```python
from build123d import *

# Parameters (mm, degrees)
BOX_W           = 18
BOX_H           = 200
BOX_DEPTH       = 137
SKETCH001_W     = 18
SKETCH001_H     = 137
POCKET001_DEPTH = 5
SKETCH003_R     = 1.55
HOLE_DEPTH      = 13.001


with BuildPart() as body002:
    # Box → Box (new body)
    with BuildSketch(Plane.XY):
        with Locations((9, 100)):
            Rectangle(BOX_W, BOX_H)
    extrude(amount=BOX_DEPTH)

    # Sketch001 (on Face2 of BaseFeature001) → Pocket001 (cut)
    with BuildSketch(Plane.YZ.offset(18)):
        with Locations((141, 68.5)):
            Rectangle(SKETCH001_W, SKETCH001_H)
    extrude(amount=-POCKET001_DEPTH, mode=Mode.SUBTRACT)

    # Sketch003 (on Face9 of Pocket001) → Hole (cut, through all)
    with BuildSketch(Plane.YZ.offset(13)):
        with Locations((141, 97)):
            Circle(SKETCH003_R)
        with Locations((141, 57)):
            Circle(SKETCH003_R)
        with Locations((141, 17)):
            Circle(SKETCH003_R)
    extrude(amount=-HOLE_DEPTH, mode=Mode.SUBTRACT)


with BuildPart() as rightleg:
    # Part__Mirroring: instance of Body002
    add(body002.part.mirror(Plane(origin=(0, 0, 0), x_dir=(0, -1, 0), z_dir=(1, 0, 0))))


with BuildPart() as rightleg_1:
    # Part__Mirroring placement: moved
    add(rightleg.part.moved(Location((350, 0, 0))))


solid = rightleg_1.part
```
The model under review builds one solid part; all positions refer to its coordinate system, in mm. A direction names the side the tool comes from. Give positions to 0.01 mm unless a question says otherwise; leave off trailing zeros. Write each loop counter-clockwise with the first axis right and the second up, starting at its lowest first coordinate (ties: lowest second). Pieces come first, ordered by that corner, then holes. Notation, with made-up numbers: (45.25, 60) -> (67.25, 60) arc R19 cw to (67.25, 66) -> close; hole circle Ø11 at (52.25, 38.25). An arc over 180 degrees is marked (long way). Answer in a Markdown table with one row per item.
1) Tool access review of faces 1 (the flat face through (341, 200, 68)), 2 (the flat face through (337, 141, 69)): name each direction out of +Z, -Z, +X, -X, +Y, -Y from which nothing blocks a thin tool from reaching the whole face with its end or side.
Worked answers:
| item | result |
|---|---|
| face 1 | +Z, -Z, +X, -X, +Y |
| face 2 | +Z, -Z, -X |
2) Clearance check with flat-ended pins moving along their axes: P1, Ø4, axis at y = 141, z = 97, coming from the +X side; P2, Ø5, axis at y = 141, z = 17, coming from the -X side. State where each tip first meets the part, or that it passes through.
Worked answers:
| item | result |
|---|---|
| P1 | x = 350 |
| P2 | x = 337 |
3) Add section B-B on y = 137.5. State the section outline as (x, z) points, plus the area to 3 significant figures.
Worked answers:
| item | result |
|---|---|
| outline | (337, 0) -> (350, 0) -> (350, 137) -> (337, 137) -> close |
| area | 1,780 mm² |
4) For L1, parallel to Z at x = 340, y = 141; L2, parallel to Y at x = 342.75, z = 97; L3, parallel to Y at x = 334.25, z = 69, list the stretches that pass through material, from the lowest coordinate up. Write a range as [from, to].
Worked answers:
| item | result |
|---|---|
| L1 | [0, 15.45], [18.55, 55.45], [58.55, 95.45], [98.55, 137] |
| L2 | [0, 139.45], [142.55, 200] |
| L3 | [0, 132], [150, 200] |
5) Add section A-A on z = 85. State the section outline as (x, y) points.
Worked answers:
| item | result |
|---|---|
| outline | (332, 0) -> (350, 0) -> (350, 200) -> (332, 200) -> (332, 150) -> (337, 150) -> (337, 132) -> (332, 132) -> close |
